Here's how the part is built. I have some questions about the finished solid (model axes, mm). A direction names the side the tool comes from. Give positions to 0.01 mm unless a question says otherwise; leave off trailing zeros. Write each loop counter-clockwise with the first axis right and the second up, starting at its lowest first coordinate (ties: lowest second). Pieces come first, ordered by that corner, then holes. Notation, with made-up numbers: (-5.5, 78.5) -> (18.5, 78.5) arc R16 ccw to (18.5, 85.5) -> close; hole circle Ø11 at (10.25, -6). An arc over 180 degrees is marked (long way). Use one line per item in the form item = value.
```python
from build123d import *

# Parameters (mm, degrees)
EXTRUDE_2_DEPTH      = 7
SKETCH_1_4_R         = 5
EXTRUDE_3_DEPTH      = 1.2
SKETCH_1_5_R         = 3
EXTRUDE_4_DEPTH      = 14
SKETCH_1_6_R         = 4.3
EXTRUDE_5_DEPTH      = 9
SKETCH_1_8_R         = 3.8
EXTRUDE_6_DEPTH      = 2
FILLET_1_R           = 1
CUT_EXTRUDE_START    = -2
SKETCH_1_10_R        = 1.6
CUT_EXTRUDE_31_DEPTH = 17
SKETCH_1_11_R        = 3
SKETCH_1_11_R_2      = 1.6
CUT_EXTRUDE_32_DEPTH = 7
CHAMFER_1_SIZE       = 0.5


with BuildPart() as part:
    # Эскиз1 → Бобышка-Вытянуть2 (new body)
    with BuildSketch(Plane.XY):
        Polygon((0, 5.773502692), (-5, 2.886751346), (-5, -2.886751346), (0, -5.773502692), (5, -2.886751346), (5, 2.886751346), align=None)
    extrude(amount=EXTRUDE_2_DEPTH)

    # Эскиз1<4> → Бобышка-Вытянуть3 (add)
    with BuildSketch(Plane.XY):
        Circle(SKETCH_1_4_R)
    extrude(amount=-EXTRUDE_3_DEPTH)

    # Эскиз1<5> → Бобышка-Вытянуть4 (add)
    with BuildSketch(Plane.XY):
        Circle(SKETCH_1_5_R)
    extrude(amount=EXTRUDE_4_DEPTH)

    # Эскиз1<6> → Бобышка-Вытянуть5 (add)
    with BuildSketch(Plane.XY):
        Circle(SKETCH_1_6_R)
    extrude(amount=EXTRUDE_5_DEPTH)

    # Эскиз1<8> → Бобышка-Вытянуть6 (add)
    with BuildSketch(Plane.XY):
        Circle(SKETCH_1_8_R)
    extrude(amount=-EXTRUDE_6_DEPTH)

    # Скругление1
    fillet_1_edges = [part.edges().sort_by_distance(p)[0] for p in [
        (-5, 0, -1.2),
    ]]
    fillet(fillet_1_edges, radius=FILLET_1_R)

    # Эскиз1<10> → Вырез-Вытянуть31 (cut, through all)
    with BuildSketch(Plane.XY.offset(CUT_EXTRUDE_START)):
        Circle(SKETCH_1_10_R)
    extrude(amount=CUT_EXTRUDE_31_DEPTH, mode=Mode.SUBTRACT)

    # Эскиз1<11> → Вырез-Вытянуть32 (cut)
    with BuildSketch(Plane.XY.offset(CUT_EXTRUDE_START)):
        Circle(SKETCH_1_11_R)
        Circle(SKETCH_1_11_R_2, mode=Mode.SUBTRACT)
    extrude(amount=CUT_EXTRUDE_32_DEPTH, mode=Mode.SUBTRACT)

    # Фаска1
    chamfer_1_edges = [part.edges().sort_by_distance(p)[0] for p in [
        (-3, 0, 14),
    ]]
    chamfer(chamfer_1_edges, length=CHAMFER_1_SIZE)


solid = part.part
```
Q1. Which directions (+Z, -Z, +X, -X, +Y, -Y) give clear straight access to the entire face, cutting with the end or side of a thin tool? Please do faces 1 (the face through (-3, -1, 9)), 2 (the face through (-3.796, 0.167, -1.594)), 3 (the face through (4.5, 2.7, 0)).
Result set:
face_1 = +Z
face_2 = -Z
face_3 = -Z, +X, +Y
Q2. I want a section at A-A, the plane z = 0.25. Write out the boundary of the cut face in (x, y).
Result set:
outline = (-5, -2.89) -> (0, -5.77) -> (5, -2.89) -> (5, 2.89) -> (0, 5.77) -> (-5, 2.89) -> close; hole circle Ø6 at (0, 0)
Q3. I want a section at B-B, the plane z = 6.25. Write out the boundary of the cut face in (x, y), and give its area (3 significant figures).
Result set:
outline = (-5, -2.89) -> (0, -5.77) -> (5, -2.89) -> (5, 2.89) -> (0, 5.77) -> (-5, 2.89) -> close; hole circle Ø3.2 at (0, 0)
area = 78.6 mm2
Q4. If I drill on line 1 along Y through (x, z) = (0, 11); line 2 along X through (y, z) = (0, 8); line 3 along Z through (x, y) = (-2, 0.5), over which ranges is the centre line in solid material (lowest first)? Write a range as from..to.
Result set:
line_1 = -3..-1.6, 1.6..3
line_2 = -4.3..-1.6, 1.6..4.3
line_3 = 5..14
Q5. Will these pins go through, and if not, where does the flat tip stop? pin 1 Ø4 at (y, z) = (3, 12) entering from -X; pin 2 Ø1 at (x, z) = (-1, 8) entering from +Y; pin 3 Ø1.2 at (x, y) = (-1, -5) entering from -Z; pin 4 Ø2.5 at (x, y) = (0, 0) entering from -Z.
Result set:
pin_1 = -2.83
pin_2 = 4.27
pin_3 = -1.07
pin_4 = through
Q6. I want a section at C-C, the plane z = 13.25. Write out the boundary of the cut face in (x, y).
Result set:
outline = circle Ø6 at (0, 0); hole circle Ø3.2 at (0, 0)
